from build123d import *

# Parameters (mm, degrees)
SKETCH1_W           = 184
SKETCH1_H           = 228
BOSS_EXTRUDE1_DEPTH = 59
SKETCH2_W           = 176
SKETCH2_H           = 220
CUT_EXTRUDE1_DEPTH  = 55
SKETCH4_R           = 4
CUT_EXTRUDE2_DEPTH  = 157.476835346
SKETCH6_R           = 12.5
CUT_EXTRUDE3_DEPTH  = 157.476835346


with BuildPart() as part:
    # Sketch1 → Boss-Extrude1 (new body)
    with BuildSketch(Plane(origin=(0, 0, 0), x_dir=(1, 0, 0), z_dir=(0, 1, 0))):
        Rectangle(SKETCH1_W, SKETCH1_H)
    extrude(amount=BOSS_EXTRUDE1_DEPTH)

    # Sketch2 → Cut-Extrude1 (cut)
    with BuildSketch(Plane(origin=(0, 59, 0), x_dir=(1, 0, 0), z_dir=(0, 1, 0))):
        Rectangle(SKETCH2_W, SKETCH2_H)
    extrude(amount=-CUT_EXTRUDE1_DEPTH, mode=Mode.SUBTRACT)

    # Sketch4 → Cut-Extrude2 (cut, through all)
    with BuildSketch(Plane(origin=(0, 4, 0), x_dir=(1, 0, 0), z_dir=(0, 1, 0))):
        with Locations(Location((-79, -95, 0), (0, 0, 270))):
            Circle(SKETCH4_R)
        with Locations(Location((-79, 95, 0), (0, 0, 270))):
            Circle(SKETCH4_R)
        with Locations(Location((79, -95, 0), (0, 0, 270))):
            Circle(SKETCH4_R)
        with Locations(Location((79, 95, 0), (0, 0, 270))):
            Circle(SKETCH4_R)
        with BuildLine():
            Line((-77.5, 70), (-77.5, 62))
            ThreePointArc((-77.5, 62), (-79, 60.5), (-80.5, 62))
            Line((-80.5, 62), (-80.5, 70))
            ThreePointArc((-80.5, 70), (-79, 71.5), (-77.5, 70))
        make_face()
        with BuildLine():
            Line((-77.5, -62), (-77.5, -70))
            ThreePointArc((-77.5, -70), (-79, -71.5), (-80.5, -70))
            Line((-80.5, -70), (-80.5, -62))
            ThreePointArc((-80.5, -62), (-79, -60.5), (-77.5, -62))
        make_face()
        with BuildLine():
            Line((80.5, -62), (80.5, -70))
            ThreePointArc((80.5, -70), (79, -71.5), (77.5, -70))
            Line((77.5, -70), (77.5, -62))
            ThreePointArc((77.5, -62), (79, -60.5), (80.5, -62))
        make_face()
        with BuildLine():
            Line((79, 70), (79, 62))
            ThreePointArc((79, 62), (77.5, 60.5), (76, 62))
            Line((76, 62), (76, 70))
            ThreePointArc((76, 70), (77.5, 71.5), (79, 70))
        make_face()
    extrude(amount=-CUT_EXTRUDE2_DEPTH, mode=Mode.SUBTRACT)

    # Sketch6 → Cut-Extrude3 (cut, through all)
    with BuildSketch(Plane(origin=(0, 4, 0), x_dir=(1, 0, 0), z_dir=(0, 1, 0))):
        with Locations(Location((-60, 0, 0), (0, 0, 270))):
            Circle(SKETCH6_R)
        with Locations(Location((0, -80, 0), (0, 0, 270))):
            Circle(SKETCH6_R)
    extrude(amount=-CUT_EXTRUDE3_DEPTH, mode=Mode.SUBTRACT)


solid = part.part
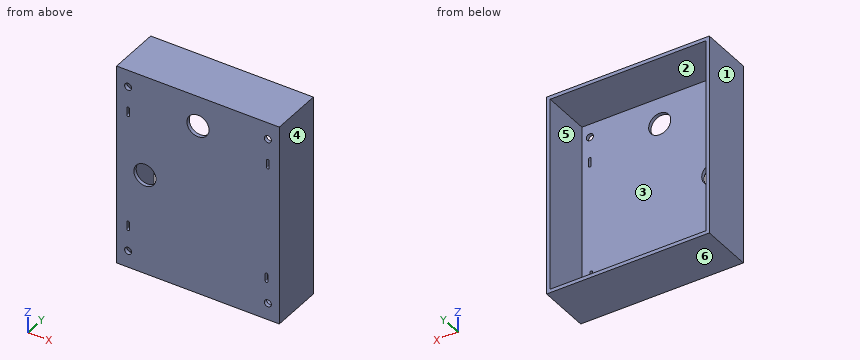
Read the model definition and answer for the solid it produces. Units are mm, in the model's axes. Face numbers are marked on the shaded views. A direction names the side the tool comes from. Coordinates: 2 decimals unless noted, no trailing zeros. Loops run counter-clockwise (first coordinate to the right, second up) from the corner with the lowest first, then second, coordinate; pieces in that order, holes last. Notation, with made-up numbers: (-29.5, 75) - (-9.5, 75) arc R32 cw to (-9.5, 103) - close; hole circle Ø3 at (-9.5, 71). An arc over 180 degrees is marked (long way). Answer in a Markdown table with one row per item.
Q1. Find section A-A on z = 0. Write down the section's boundary in (x, y).
Here are the results:
| item | result |
|---|---|
| outline | (-92, 0) - (-72.5, 0) - (-72.5, 4) - (-88, 4) - (-88, 59) - (-92, 59) - close; (-47.5, 0) - (92, 0) - (92, 59) - (88, 59) - (88, 4) - (-47.5, 4) - close |
Q2. Find section D-D on z = -95. Write down the section's boundary in (x, y), plus the area to 3 significant figures.
Here are the results:
| item | result |
|---|---|
| outline | (-92, 0) - (-83, 0) - (-83, 4) - (-88, 4) - (-88, 59) - (-92, 59) - close; (-75, 0) - (75, 0) - (75, 4) - (-75, 4) - close; (83, 0) - (92, 0) - (92, 59) - (88, 59) - (88, 4) - (83, 4) - close |
| area | 1,110 mm^2 |
Q3. Find section B-B on x = -7.5. Write down the section's boundary in (y, z), plus the area to 3 significant figures.
Here are the results:
| item | result |
|---|---|
| outline | (0, -114) - (59, -114) - (59, -110) - (4, -110) - (4, 70) - (0, 70) - close; (0, 90) - (4, 90) - (4, 110) - (59, 110) - (59, 114) - (0, 114) - close |
| area | 1,270 mm^2 |
Q4. Find section C-C on y = 40. Write down the section's boundary in (x, z), plus the area to 3 significant figures.
Here are the results:
| item | result |
|---|---|
| outline | (-92, -114) - (92, -114) - (92, 114) - (-92, 114) - close; hole (-88, -110) - (88, -110) - (88, 110) - (-88, 110) - close |
| area | 3,230 mm^2 |
Q5. Straight lines are drawn through the part: line 1 along X through (y, z) = (0.9, -95); line 2 along Z through (x, y) = (-58, 41.5); line 3 along X through (y, z) = (29, -31). For each, find the intervals that lie inside material, in ascending order. Write a range as [from, to].
Here are the results:
| item | result |
|---|---|
| line 1 | x = [-92, -83], [-75, 75], [83, 92] |
| line 2 | z = [-114, -110], [110, 114] |
| line 3 | x = [-92, -88], [88, 92] |
Q6. Given P1, Ø10.5, axis at x = -79, z = -95, coming from the +Y side, flat-ended and moving along its own axis, determine where the tip first touches the part or whether it passes through.
Here are the results:
| item | result |
|---|---|
| P1 | stops at y = 4 |
Q7. The mould has two halves that part along X. Classify the marked faces 1, 2, 3 and 4: pulls with the +X half, pulls with the -X half, needs draft (parallel to the pull), parting line crosses it, or undercut.
Here are the results:
| item | result |
|---|---|
| face 1 | pulls with the -X half |
| face 2 | undercut |
| face 3 | undercut |
| face 4 | pulls with the +X half |
Q8. For the marked faces 5 and 6, determine the directions among +Z, -Z, +X, -X, +Y, -Y from which every point of the face is accessible in a straight line to the end or side of a thin tool.
Here are the results:
| item | result |
|---|---|
| face 5 | +Y |
| face 6 | -Z, +X, -X, +Y, -Y |
